Here's how the part is built. I have some questions about the finished solid (model axes, mm). A direction names the side the tool comes from. Round coordinates to 2 decimals unless told otherwise and drop trailing zeros. Write each loop counter-clockwise with the first axis right and the second up, starting at its lowest first coordinate (ties: lowest second). Pieces come first, ordered by that corner, then holes. Notation, with made-up numbers: (56, 9) - (78, 9) arc R27 ccw to (78, 38) - close; hole circle Ø11 at (-4, 89). An arc over 180 degrees is marked (long way). Use one line per item in the form item = value. Start each with the question number.
1. I want a section at C-C, the plane z = 17.5. List the corners of the cut face in (x, y) for me.
2. Will these pins go through, and if not, where does the flat tip stop? pin 1 (1.3 mm diameter, centred on y = 11, z = -26, fed in from +X); pin 2 (1.2 mm diameter, centred on y = 4.75, z = -18.84, fed in from +X); pin 3 (12 mm diameter, centred on x = -9, y = 12, fed in from -Z).
3. I want a section at B-B, the plane x = -23. List the corners of the cut face in (y, z) for me, plus the area to 3 significant figures.
4. If I drill on line 1 along X through (y, z) = (8.25, 30); line 2 along Z through (x, y) = (-48.5, 14.75); line 3 along Z through (x, y) = (11, 14.25), over which ranges is the centre line in solid material (lowest first)?
5. I want a section at A-A, the plane y = 10. List the corners of the cut face in (x, z) for me.
6. We'd pull the mould along X, two halves only. Please class faces 6 (the flat face through (-16.77, 10, 32)), 7 (the flat face through (-53.57, 13, 6)), 8 (the flat face through (5.5, 9.9, 38.414)): +X half, -X half, draft (parallel to the pull), parting line (faces both ways), or undercut.
7. I want a section at D-D, the plane y = 4.75. List the corners of the cut face in (x, z) for me.
8. Which directions (+Z, -Z, +X, -X, +Y, -Y) give clear straight access to the entire face, cutting with the end or side of a thin tool? Please do faces 1 (the flat face through (-46, 10, -26.586)), 2 (the flat face through (-33, 10, -26.586)), 3 (the flat face through (-13.27, 10, 32)), 4 (the cylindrical face through (-14.996, 4.794, -17.837)), 5 (the flat face through (-49.27, 10, 7)).
```python
from build123d import *

# Parameters (mm, degrees)
SALIENTE_EXTRUIR1_DEPTH = 20
CROQUIS2_R              = 4
CORTAR_EXTRUIR1_DEPTH   = 1.2
CROQUIS3_R              = 1
CORTAR_EXTRUIR3_DEPTH   = 1.8
CROQUIS4_R              = 1
CORTAR_EXTRUIR4_DEPTH   = 3.5
CROQUIS7_R              = 1
CORTAR_EXTRUIR5_DEPTH   = 3.5
CROQUIS8_W              = 5
CROQUIS8_H              = 8
CORTAR_EXTRUIR6_DEPTH   = 3
CROQUIS9_W              = 12
CROQUIS9_H              = 2
SALIENTE_EXTRUIR2_DEPTH = 1.3
CROQUIS10_W             = 69.3
CROQUIS10_H             = 2
SALIENTE_EXTRUIR3_DEPTH = 1.3


with BuildPart() as part:
    # Croquis1 → Saliente-Extruir1 (new body)
    with BuildSketch(Plane(origin=(0, 0, 0), x_dir=(1, 0, 0), z_dir=(0, 1, 0))):
        Polygon((24.729603414, -41.414237295), (-52.270396586, -41.414237295), (-52.270396586, 26.585762705), (-13.270396586, 26.585762705), (-13.270396586, 14.585762705), (-16.770396586, 14.585762705), (-16.770396586, 23.585762705), (-49.270396586, 23.585762705), (-49.270396586, -38.414237295), (-16.770396586, -38.414237295), (-16.770396586, -26.414237295), (-13.270396586, -26.414237295), (-13.270396586, -38.414237295), (24.729603414, -38.414237295), align=None)
    extrude(amount=SALIENTE_EXTRUIR1_DEPTH)

    # Croquis2 → Cortar-Extruir1 (cut)
    with BuildSketch(Plane.XY.offset(41.414237295)):
        with Locations((4.229603414, 10)):
            Circle(CROQUIS2_R)
    extrude(amount=-CORTAR_EXTRUIR1_DEPTH, mode=Mode.SUBTRACT)

    # Croquis3 → Cortar-Extruir3 (cut)
    with BuildSketch(Plane.XY.offset(40.214237295)):
        with Locations((4.229603414, 10)):
            Circle(CROQUIS3_R)
    extrude(amount=-CORTAR_EXTRUIR3_DEPTH, mode=Mode.SUBTRACT)

    # Croquis4 → Cortar-Extruir4 (cut)
    with BuildSketch(Plane(origin=(-13.270396586, 0, 0), x_dir=(0, 0, -1), z_dir=(1, 0, 0))):
        with Locations((-30.664237295, 15.25)):
            Circle(CROQUIS4_R)
        with Locations((-30.664237295, 4.75)):
            Circle(CROQUIS4_R)
    extrude(amount=-CORTAR_EXTRUIR4_DEPTH, mode=Mode.SUBTRACT)

    # Croquis7 → Cortar-Extruir5 (cut)
    with BuildSketch(Plane(origin=(-13.270396586, 0, 0), x_dir=(0, 0, -1), z_dir=(1, 0, 0))):
        with Locations((18.835762705, 15.25)):
            Circle(CROQUIS7_R)
        with Locations((18.835762705, 4.75)):
            Circle(CROQUIS7_R)
    extrude(amount=-CORTAR_EXTRUIR5_DEPTH, mode=Mode.SUBTRACT)

    # Croquis8 → Cortar-Extruir6 (cut)
    with BuildSketch(Plane.XY.offset(-23.585762705)):
        with Locations((-37.770396586, 10)):
            Rectangle(CROQUIS8_W, CROQUIS8_H)
    extrude(amount=-CORTAR_EXTRUIR6_DEPTH, mode=Mode.SUBTRACT)

    # Croquis9 → Saliente-Extruir2 (add)
    with BuildSketch(Plane(origin=(0, 0, -26.585762705), x_dir=(-1, 0, 0), z_dir=(0, 0, -1))):
        with Locations((46.270396586, 7)):
            Rectangle(CROQUIS9_W, CROQUIS9_H)
        with Locations((46.270396586, 13)):
            Rectangle(CROQUIS9_W, CROQUIS9_H)
    extrude(amount=SALIENTE_EXTRUIR2_DEPTH)

    # Croquis10 → Saliente-Extruir3 (add)
    with BuildSketch(Plane.ZY.offset(52.270396586)):
        with Locations((6.764237295, 13)):
            Rectangle(CROQUIS10_W, CROQUIS10_H)
        with Locations((6.764237295, 7)):
            Rectangle(CROQUIS10_W, CROQUIS10_H)
    extrude(amount=SALIENTE_EXTRUIR3_DEPTH)


solid = part.part
```
Model answer:
q1.outline = (-53.57, 6) - (-52.27, 6) - (-52.27, 0) - (-49.27, 0) - (-49.27, 20) - (-52.27, 20) - (-52.27, 14) - (-53.57, 14) - (-53.57, 12) - (-52.27, 12) - (-52.27, 8) - (-53.57, 8) - close
q2.pin_1 = -13.27
q2.pin_2 = -49.27
q2.pin_3 = -26.59
q3.outline = (0, -26.59) - (20, -26.59) - (20, -23.59) - (0, -23.59) - close; (0, 38.41) - (20, 38.41) - (20, 41.41) - (0, 41.41) - close
q3.area = 120 mm2
q4.line_1 = -52.27 to -49.27, -16.77 to -13.27
q4.line_2 = -26.59 to -23.59, 38.41 to 41.41
q4.line_3 = 38.41 to 41.41
q5.outline = (-52.27, -26.59) - (-40.27, -26.59) - (-40.27, -23.59) - (-49.27, -23.59) - (-49.27, 38.41) - (-16.77, 38.41) - (-16.77, 26.41) - (-13.27, 26.41) - (-13.27, 38.41) - (3.23, 38.41) - (3.23, 40.21) - (0.23, 40.21) - (0.23, 41.41) - (-52.27, 41.41) - close; (-35.27, -26.59) - (-13.27, -26.59) - (-13.27, -14.59) - (-16.77, -14.59) - (-16.77, -23.59) - (-35.27, -23.59) - close; (5.23, 38.41) - (24.73, 38.41) - (24.73, 41.41) - (8.23, 41.41) - (8.23, 40.21) - (5.23, 40.21) - close
q6.face_6 = undercut
q6.face_7 = -X half
q6.face_8 = draft
q7.outline = (-52.27, -26.59) - (-13.27, -26.59) - (-13.27, -19.84) - (-16.77, -19.84) - (-16.77, -23.59) - (-49.27, -23.59) - (-49.27, 38.41) - (-16.77, 38.41) - (-16.77, 31.66) - (-13.27, 31.66) - (-13.27, 38.41) - (24.73, 38.41) - (24.73, 41.41) - (-52.27, 41.41) - close; (-16.77, -17.84) - (-13.27, -17.84) - (-13.27, -14.59) - (-16.77, -14.59) - close; (-16.77, 26.41) - (-13.27, 26.41) - (-13.27, 29.66) - (-16.77, 29.66) - close
q8.face_1 = -Z, +X, -X
q8.face_2 = -Z, +X
q8.face_3 = -Z, +X, +Y, -Y
q8.face_4 = +X
q8.face_5 = +Y, -Y
